Could you check a few things on this drawing? It's one solid part, dimensions in mm from its lowest x, y, z. A direction names the side the tool comes from. Coordinates: 2 decimals unless noted, no trailing zeros. Write each loop counter-clockwise with the first axis right and the second up, starting at its lowest first coordinate (ties: lowest second). Pieces come first, ordered by that corner, then holes.
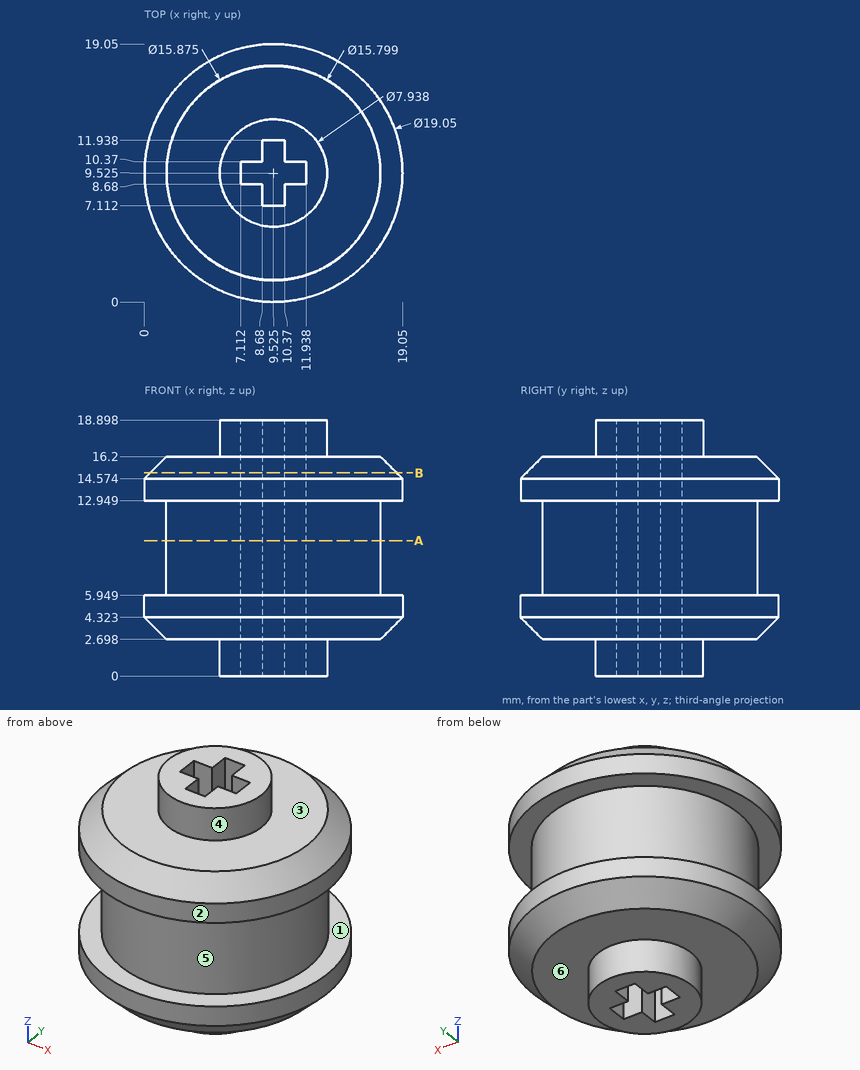
1) Imagine slicing it at B-B on z = 15. Please give me the cut outline in (x, y) (1 decimal), then the cut area to 3 significant figures.
Values follow:
outline: circle Ø18.2 at (9.5, 9.5); hole (7.1, 8.7) - (8.7, 8.7) - (8.7, 7.1) - (10.4, 7.1) - (10.4, 8.7) - (11.9, 8.7) - (11.9, 10.4) - (10.4, 10.4) - (10.4, 11.9) - (8.7, 11.9) - (8.7, 10.4) - (7.1, 10.4) - close
area: 247 mm2
2) Imagine slicing it at A-A on z = 10. Please give me the cut outline in (x, y) (1 decimal).
Values follow:
outline: circle Ø15.9 at (9.5, 9.5); hole (7.1, 8.7) - (8.7, 8.7) - (8.7, 7.1) - (10.4, 7.1) - (10.4, 8.7) - (11.9, 8.7) - (11.9, 10.4) - (10.4, 10.4) - (10.4, 11.9) - (8.7, 11.9) - (8.7, 10.4) - (7.1, 10.4) - close
3) Will these pins go through, and if not, where does the flat tip stop? pin 1 (6 mm diameter, centred on x = 4, z = 3, fed in from +Y); pin 2 (0.5 mm diameter, centred on x = 9, z = 10, fed in from -Y); pin 3 (0.5 mm diameter, centred on y = 7.5, z = 13.5, fed in from +X); pin 4 (3 mm diameter, centred on y = 8.5, z = 5.5, fed in from -X).
Values follow:
pin 1: stops at y = 18.62
pin 2: stops at y = 1.59
pin 3: stops at x = 18.88
pin 4: stops at x = 0
4) I need wall thicknesses on probe 1 along Z at (x, y) = (2.5, 6.25); probe 2 along X at (y, z) = (9.5, 4.5); probe 3 along X at (y, z) = (11, 10.25) (1 decimal). Which ranges of each line are inside material? Lowest first, please.
Values follow:
probe 1: z = 2.7 to 16.2
probe 2: x = 0 to 7.11, 11.94 to 19.05
probe 3: x = 1.7 to 8.7, 10.4 to 17.3
5) We'd pull the mould along Z, two halves only. Please class the marked faces 1, 2 and 3: pulls with the +Z half, pulls with the -Z half, needs draft (parallel to the pull), parting line crosses it, or undercut.
Values follow:
face 1: undercut
face 2: needs draft
face 3: pulls with the +Z half
6) On a 3-axis mill with a long thin cutter (end or side, diameter ignored), from which of +Z, -Z, +X, -X, +Y, -Y can I reach the whole of each face in a straight line? I mean the marked faces 4, 5 and 6. Say none if no direction works.
Values follow:
face 4: +Z
face 5: none
face 6: -Z
